Read the model definition and answer for the solid it produces. Units are mm, in the model's axes. Face numbers are marked on the shaded views. A direction names the side the tool comes from. Give positions to 0.01 mm unless a question says otherwise; leave off trailing zeros. Write each loop counter-clockwise with the first axis right and the second up, starting at its lowest first coordinate (ties: lowest second). Pieces come first, ordered by that corner, then holes. Notation, with made-up numbers: (-40, 19) - (-21, 19) arc R20 ccw to (-21, 45) - close; hole circle Ø3 at (43.5, 64.25). An arc over 180 degrees is marked (long way). Answer as CSV lines item,"result".
```python
from build123d import *

# Parameters (mm, degrees)
F0_W          = 30
F0_H          = 20
F1_DEPTH      = 10
F1_DEPTH_BACK = 10
F2_SIZE       = 5
F3_T          = -1


with BuildPart() as f1:
    # F0 (on Front) → F1 (new body, two sides)
    with BuildSketch(Plane.XZ) as f1_sk:
        Rectangle(F0_W, F0_H)
    extrude(amount=-F1_DEPTH)
    extrude(f1_sk.sketch, amount=F1_DEPTH_BACK)

    # F2
    f2_edges = [f1.edges().sort_by_distance(p)[0] for p in [
        (-15, 0, 10),
    ]]
    chamfer(f2_edges, length=F2_SIZE)

    # F3
    f3_openings = [f1.faces().sort_by_distance(p)[0] for p in [
        (2.5, 0, 10),
        (-12.5, 0, 7.5),
    ]]
    offset(amount=F3_T, openings=f3_openings)


solid = f1.part
```
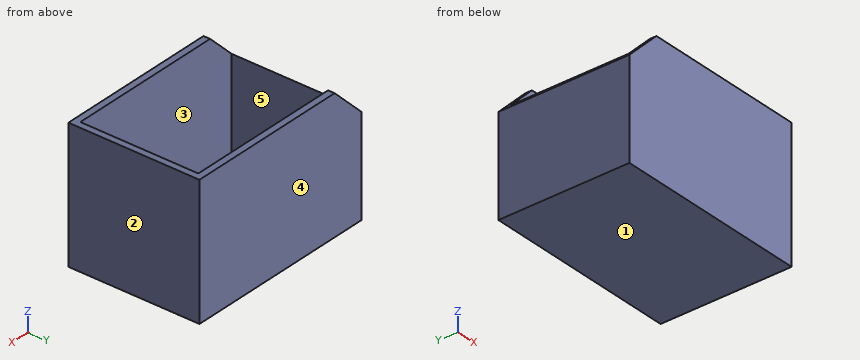
(1) A cutting plane is placed at B-B (y = 1). Write down the section's boundary in (x, z).
Worked out:
outline,"(-15, -10) - (15, -10) - (15, 10) - (14, 10) - (14, -9) - (-14, -9) - (-14, 6) - (-15, 5) - close"
(2) A cutting plane is placed at C-C (x = 1.25). Write down the section's boundary in (y, z).
Worked out:
outline,"(-10, -10) - (10, -10) - (10, 10) - (9, 10) - (9, -9) - (-9, -9) - (-9, 10) - (-10, 10) - close"
(3) For the marked faces 4 and 5, determine the directions among +Z, -Z, +X, -X, +Y, -Y from which every point of the face is accessible in a straight line to the end or side of a thin tool.
Worked out:
face 4,"+Z, -Z, +X, -X, +Y"
face 5,"+Z"
(4) This flat-tipped pin is pushed along its axis until it touches: P1, Ø5.5, axis at x = -2, y = -3, coming from the +Z side. Where does it stop, or does it pass through?
Worked out:
P1,"stops at z = -9"
(5) Find the intervals of material crossed by L1, parallel to X at y = 1.75, z = -1.25; L2, parallel to Y at x = 9.75, z = -8.5; L3, parallel to Z at x = 4.75, y = 6.75, in increasing order.
Worked out:
L1,"x = -15 to -14, 14 to 15"
L2,"y = -10 to -9, 9 to 10"
L3,"z = -10 to -9"
(6) The mould has two halves that part along X. Classify the marked faces 1, 2 and 3: +X half, -X half, draft (parallel to the pull), parting line (faces both ways), or undercut.
Worked out:
face 1,"draft"
face 2,"+X half"
face 3,"undercut"
(7) A cutting plane is placed at A-A (z = -8.25). Write down the section's boundary in (x, y), and give its area (3 significant figures).
Worked out:
outline,"(-15, -10) - (15, -10) - (15, 10) - (-15, 10) - close; hole (-14, -9) - (14, -9) - (14, 9) - (-14, 9) - close"
area,"96.0 mm^2"
